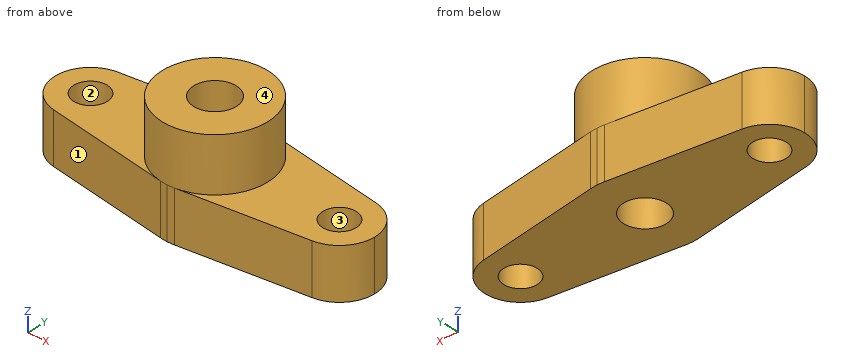
from build123d import *

# Parameters (mm, degrees)
SKETCH_1_W             = 32
SKETCH_1_H             = 10.4
SKETCH_1_R             = 0.5
EXTRUDE_1_DEPTH        = 5
SKETCH_2_R             = 5.2
SKETCH_2_R_2           = 0.5
EXTRUDE_2_DEPTH        = 5.3
CUT_EXTRUDE_1_DEPTH    = 5.3
HOLE_WIZARD_M4_1_D     = 3.3
HOLE_WIZARD_M4_1_DEPTH = 10.1
HOLE_WIZARD_M4_1_TIP   = 0.991420021
HOLE_WIZARD_M5_1_D     = 4.2
HOLE_WIZARD_M5_1_DEPTH = 22.4
HOLE_WIZARD_M5_1_TIP   = 1.2618073


with BuildPart() as part:
    # 草图1 → 凸台-拉伸1 (new body)
    with BuildSketch(Plane.XY):
        Rectangle(SKETCH_1_W, SKETCH_1_H)
        with Locations((-12.5, 0)):
            Circle(SKETCH_1_R, mode=Mode.SUBTRACT)
        with Locations((12.5, 0)):
            Circle(SKETCH_1_R, mode=Mode.SUBTRACT)
        Circle(SKETCH_1_R, mode=Mode.SUBTRACT)
    extrude(amount=EXTRUDE_1_DEPTH)

    # 草图2 → 凸台-拉伸2 (add)
    with BuildSketch(Plane.XY.offset(5)):
        Circle(SKETCH_2_R)
        Circle(SKETCH_2_R_2, mode=Mode.SUBTRACT)
    extrude(amount=EXTRUDE_2_DEPTH)

    # 草图3 → 切除-拉伸1 (cut)
    with BuildSketch(Plane.XY.offset(5)):
        with BuildLine():
            Line((-12.976, 3.46748093), (-0.7072, 5.151685953))
            ThreePointArc((-0.7072, 5.151685953), (-0.354424212, 5.187907428), (0, 5.2))
            Line((0, 5.2), (-16, 5.2))
            Line((-16, 5.2), (-16, 0))
            ThreePointArc((-16, 0), (-15.137802115, 2.300434742), (-12.976, 3.46748093))
        make_face()
        with BuildLine():
            ThreePointArc((0, -5.2), (-0.354424212, -5.187907428), (-0.7072, -5.151685953))
            Line((-0.7072, -5.151685953), (-12.976, -3.46748093))
            ThreePointArc((-12.976, -3.46748093), (-15.137802115, -2.300434742), (-16, 0))
            Line((-16, 0), (-16, -5.2))
            Line((-16, -5.2), (0, -5.2))
        make_face()
        with BuildLine():
            ThreePointArc((0.7072, -5.151685953), (0.354424212, -5.187907428), (0, -5.2))
            Line((0, -5.2), (16, -5.2))
            Line((16, -5.2), (16, 0))
            ThreePointArc((16, 0), (15.137802115, -2.300434742), (12.976, -3.46748093))
            Line((12.976, -3.46748093), (0.7072, -5.151685953))
        make_face()
        with BuildLine():
            Line((16, 5.2), (0, 5.2))
            ThreePointArc((0, 5.2), (0.354424212, 5.187907428), (0.7072, 5.151685953))
            Line((0.7072, 5.151685953), (12.976, 3.46748093))
            ThreePointArc((12.976, 3.46748093), (15.137802115, 2.300434742), (16, 0))
            Line((16, 0), (16, 5.2))
        make_face()
    extrude(amount=-CUT_EXTRUDE_1_DEPTH, mode=Mode.SUBTRACT)

    # M4 螺纹孔1
    with Locations(Plane.XY.offset(5)):
        with Locations((-12.5, 0), (12.5, 0)):
            Hole(HOLE_WIZARD_M4_1_D / 2, depth=HOLE_WIZARD_M4_1_DEPTH)
            with Locations((0, 0, -(HOLE_WIZARD_M4_1_DEPTH + HOLE_WIZARD_M4_1_TIP / 2))):  # 118° drill point
                Cone(0, HOLE_WIZARD_M4_1_D / 2, HOLE_WIZARD_M4_1_TIP, mode=Mode.SUBTRACT)

    # M5 螺纹孔1
    with Locations(Plane.XY.offset(10.3)):
        with Locations((0, 0)):
            Hole(HOLE_WIZARD_M5_1_D / 2, depth=HOLE_WIZARD_M5_1_DEPTH)
            with Locations((0, 0, -(HOLE_WIZARD_M5_1_DEPTH + HOLE_WIZARD_M5_1_TIP / 2))):  # 118° drill point
                Cone(0, HOLE_WIZARD_M5_1_D / 2, HOLE_WIZARD_M5_1_TIP, mode=Mode.SUBTRACT)


solid = part.part
Can you work these out from the model? Positions are in its coordinate system, mm. Face numbers are marked on the shaded views. Give positions to 0.01 mm unless a question says otherwise; leave off trailing zeros. Loops run counter-clockwise (first coordinate to the right, second up) from the corner with the lowest first, then second, coordinate; pieces in that order, holes last. Notation, with made-up numbers: (58.25, -3) -> (85.25, -3) arc R16 ccw to (85.25, 3) -> close; hole circle Ø9 at (88.5, -6.5). An arc over 180 degrees is marked (long way). Write item = value, one per line.
1) Will these pins go through, and if not, where does the flat tip stop? pin 1 (5 mm diameter, centred on x = 3, z = 6.5, fed in from +Y); pin 2 (2.5 mm diameter, centred on x = 12.5, y = 0, fed in from +Z).
Check result:
pin_1 = 5.18
pin_2 = through
2) Suppose I cut it at D-D on z = 7.25. Write out the boundary of the cut face in (x, y).
Check result:
outline = circle Ø10.4 at (0, 0); hole circle Ø4.2 at (0, 0)
3) Suppose I cut it at C-C on x = 12.5. Write out the boundary of the cut face in (y, z).
Check result:
outline = (-3.53, 0) -> (-1.65, 0) -> (-1.65, 5) -> (-3.53, 5) -> close; (1.65, 0) -> (3.53, 0) -> (3.53, 5) -> (1.65, 5) -> close
4) Thinking about a two-plate mould opening in Y: for the marked faces 1, 2, 3 and 4, which applies, released by +Y, released by -Y, zero draft, split by the parting line, or undercut?
Check result:
face_1 = released by -Y
face_2 = undercut
face_3 = undercut
face_4 = zero draft
5) Suppose I cut it at B-B on z = 1.5. Write out the boundary of the cut face in (x, y).
Check result:
outline = (-12.98, -3.47) -> (-0.71, -5.15) arc R5.2 ccw to (0.71, -5.15) -> (12.98, -3.47) arc R3.5 ccw to (12.98, 3.47) -> (0.71, 5.15) arc R5.2 ccw to (-0.71, 5.15) -> (-12.98, 3.47) arc R3.5 ccw to start; hole circle Ø3.3 at (-12.5, 0); hole circle Ø4.2 at (0, 0); hole circle Ø3.3 at (12.5, 0)
6) Suppose I cut it at A-A on y = 0.5. Write out the boundary of the cut face in (x, z).
Check result:
outline = (-15.96, 0) -> (-14.07, 0) -> (-14.07, 5) -> (-15.96, 5) -> close; (-10.93, 0) -> (-2.04, 0) -> (-2.04, 10.3) -> (-5.18, 10.3) -> (-5.18, 5) -> (-10.93, 5) -> close; (2.04, 0) -> (10.93, 0) -> (10.93, 5) -> (5.18, 5) -> (5.18, 10.3) -> (2.04, 10.3) -> close; (14.07, 0) -> (15.96, 0) -> (15.96, 5) -> (14.07, 5) -> close
7) I need wall thicknesses on L1, parallel to X at y = 0.5, z = 1.25; L2, parallel to Y at x = 0, z = 3; L3, parallel to X at y = 1.5, z = 2.75. Which ranges of each line are inside material? Lowest first, please. Write a range as from..to.
Check result:
L1 = -15.96..-14.07, -10.93..-2.04, 2.04..10.93, 14.07..15.96
L2 = -5.2..-2.1, 2.1..5.2
L3 = -15.66..-13.19, -11.81..-1.47, 1.47..11.81, 13.19..15.66
